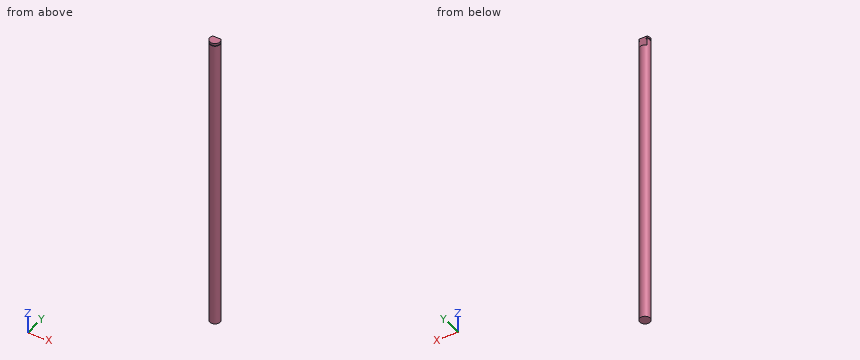
from build123d import *

# Parameters (mm, degrees)
SKETCH1_R           = 4
BOSS_EXTRUDE1_DEPTH = 325
CUT_EXTRUDE1_DEPTH  = 7.5
SKETCH3_R           = 4
SKETCH3_R_2         = 3.5
CUT_EXTRUDE2_DEPTH  = 1
SKETCH5_R           = 4
CUT_EXTRUDE3_DEPTH  = 65
SKETCH6_R           = 4
BOSS_EXTRUDE2_DEPTH = 13
SKETCH7_R           = 4
BOSS_EXTRUDE3_DEPTH = 10
SKETCH8_R           = 4
BOSS_EXTRUDE4_DEPTH = 40
SKETCH9_R           = 4
CUT_EXTRUDE4_DEPTH  = 30
SKETCH10_R          = 4
CUT_EXTRUDE5_DEPTH  = 61


with BuildPart() as part:
    # Sketch1 → Boss-Extrude1 (new body)
    with BuildSketch(Plane.XY):
        Circle(SKETCH1_R)
    extrude(amount=BOSS_EXTRUDE1_DEPTH)

    # Sketch2 → Cut-Extrude1 (cut)
    with BuildSketch(Plane.XY.offset(325)):
        with BuildLine():
            Line((3.122498999, 2.5), (-3.122498999, 2.5))
            ThreePointArc((-3.122498999, 2.5), (0, 4), (3.122498999, 2.5))
        make_face()
    extrude(amount=-CUT_EXTRUDE1_DEPTH, mode=Mode.SUBTRACT)

    # Sketch3 → Cut-Extrude2 (cut)
    with BuildSketch(Plane.XY.offset(323.75)):
        Circle(SKETCH3_R)
        Circle(SKETCH3_R_2, mode=Mode.SUBTRACT)
    extrude(amount=-CUT_EXTRUDE2_DEPTH, mode=Mode.SUBTRACT)

    # Sketch5 → Cut-Extrude3 (cut)
    with BuildSketch(Plane(origin=(0, 0, 0), x_dir=(-1, 0, 0), z_dir=(0, 0, -1))):
        Circle(SKETCH5_R)
    extrude(amount=-CUT_EXTRUDE3_DEPTH, mode=Mode.SUBTRACT)

    # Sketch6 → Boss-Extrude2 (add)
    with BuildSketch(Plane(origin=(0, 0, 65), x_dir=(-1, 0, 0), z_dir=(0, 0, -1))):
        Circle(SKETCH6_R)
    extrude(amount=BOSS_EXTRUDE2_DEPTH)

    # Sketch7 → Boss-Extrude3 (add)
    with BuildSketch(Plane(origin=(0, 0, 52), x_dir=(-1, 0, 0), z_dir=(0, 0, -1))):
        Circle(SKETCH7_R)
    extrude(amount=BOSS_EXTRUDE3_DEPTH)

    # Sketch8 → Boss-Extrude4 (add)
    with BuildSketch(Plane(origin=(0, 0, 42), x_dir=(-1, 0, 0), z_dir=(0, 0, -1))):
        Circle(SKETCH8_R)
    extrude(amount=BOSS_EXTRUDE4_DEPTH)

    # Sketch9 → Cut-Extrude4 (cut)
    with BuildSketch(Plane(origin=(0, 0, 2), x_dir=(-1, 0, 0), z_dir=(0, 0, -1))):
        Circle(SKETCH9_R)
    extrude(amount=-CUT_EXTRUDE4_DEPTH, mode=Mode.SUBTRACT)

    # Sketch10 → Cut-Extrude5 (cut)
    with BuildSketch(Plane(origin=(0, 0, 32), x_dir=(-1, 0, 0), z_dir=(0, 0, -1))):
        Circle(SKETCH10_R)
    extrude(amount=-CUT_EXTRUDE5_DEPTH, mode=Mode.SUBTRACT)


solid = part.part
The listing builds one solid part. Answer for the finished solid, in the listing's coordinates (mm). Give positions to 0.01 mm unless a question says otherwise; leave off trailing zeros. Write each loop counter-clockwise with the first axis right and the second up, starting at its lowest first coordinate (ties: lowest second). Pieces come first, ordered by that corner, then holes.
Item 1: Section A-A, the plane x = 1 is taken. Write down the section's boundary in (y, z), plus the area to 3 significant figures.
Item 2: Find the intervals of material crossed by line 1 along Z through (x, y) = (3.5, -1.5); line 2 along X through (y, z) = (0.25, 164); line 3 along Y through (x, z) = (-2, 232), in increasing order.
Item 3: Section B-B, the plane z = 220 is taken. Write down the section's boundary in (x, y), plus the area to 3 significant figures.
Item 4: Flat-ended cylindrical pins translate along their axes: P1, Ø1, axis at y = 3, z = 140.5, coming from the -X side; P2, Ø1.6, axis at x = 0.5, y = 3.5, coming from the +Z side; P3, Ø1.5, axis at x = -2.5, z = 163.5, coming from the +Y side. Find the tip coordinate at first contact, or state that the pin passes through.
Completed:
1. outline: (-3.87, 93) - (3.87, 93) - (3.87, 317.5) - (2.5, 317.5) - (2.5, 325) - (-3.87, 325) - (-3.87, 323.75) - (-3.35, 323.75) - (-3.35, 322.75) - (-3.87, 322.75) - close
1. area: 1,790 mm2
2. line 1: z = 93 to 322.75, 323.75 to 325
2. line 2: x = -3.99 to 3.99
2. line 3: y = -3.46 to 3.46
3. outline: circle Ø8 at (0, 0)
3. area: 50.3 mm2
4. P1: stops at x = -3.12
4. P2: stops at z = 317.5
4. P3: stops at y = 3.6
